The listing builds one solid part. Answer for the finished solid, in the listing's coordinates (mm). Face numbers are marked on the shaded views. A direction names the side the tool comes from. Round coordinates to 2 decimals unless told otherwise and drop trailing zeros. Write each loop counter-clockwise with the first axis right and the second up, starting at its lowest first coordinate (ties: lowest second). Pieces come first, ordered by that corner, then holes. Notation, with made-up numbers: (56, 64) - (61, 64) arc R15 cw to (61, 72) - close; hole circle Ø6 at (-27, 43). An arc over 180 degrees is marked (long way). Use a Markdown table: item, result. Add a question column.
1) A cutting plane is placed at C-C (x = 21). Give the vertices of the cut face in (y, z), then the cut area to 3 significant figures.
2) Each of these flat-tipped pins is pushed along its axis until it touches: P1, Ø2, axis at y = 8, z = -25, coming from the -X side; P2, Ø0.8, axis at y = 8, z = -25, coming from the +X side; P3, Ø6, axis at y = 9.5, z = -23, coming from the -X side. Where does it stop, or does it pass through?
3) Find the intervals of material crossed by probe 1 along Z at (x, y) = (12, 11); probe 2 along X at (y, z) = (10.75, -12); probe 3 along Z at (x, y) = (36.5, 10.75), in increasing order. Write a range as from..to.
4) A cutting plane is placed at B-B (x = 28). Give the vertices of the cut face in (y, z), then the cut area to 3 significant figures.
5) Determine the mould class of the marked faces 4, 5 and 6 for opening direction Z: +Z half, -Z half, draft (parallel to the pull), parting line (faces both ways), or undercut.
6) A cutting plane is placed at D-D (x = -3). Give the vertices of the cut face in (y, z), then the cut area to 3 significant figures.
7) A tool of negligible diameter and unlimited length cuts with its end or side. For the marked faces 1, 2 and 3, from which of +Z, -Z, +X, -X, +Y, -Y can it reach the whole face along a straight path? Write none if from no direction.
8) A cutting plane is placed at A-A (x = 8.5). Give the vertices of the cut face in (y, z), then the cut area to 3 significant figures.
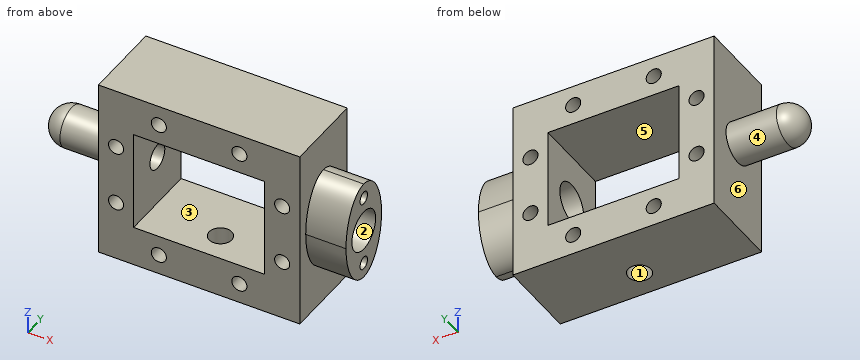
Autodesk Inventor part; units mm, degrees
ref_plane "YZ Plane" through (0, 0, 0) normal (1, 0, 0) x (0, 1, 0)
ref_plane "XZ Plane" through (0, 0, 0) normal (0, 1, 0) x (-1, 0, 0)
ref_plane "XY Plane" through (0, 0, 0) normal (0, 0, 1) x (1, 0, 0)
sketch "Sketch1" plane through (0, 0, 0) normal (0, 1, 0) x (-1, 0, 0)
  line L0 (0, 0) -> (-40, 0)
  line L1 (-40, 0) -> (-40, -36)
  line L2 (-40, -36) -> (0, -36)
  line L3 (0, -36) -> (0, 0)
  line L4 (-7, -28) -> (-33, -28)
  line L5 (-33, -28) -> (-33, -8)
  line L6 (-33, -8) -> (-7, -8)
  line L7 (-7, -8) -> (-7, -28)
  dimension "d0" = 40
  dimension "d1" = 36
  dimension "d2" = 26
extrude "Extrusion1" add sketch "Sketch1" along normal blind 16
sketch "Sketch2" plane through (40, 0, 0) normal (1, 0, 0) x (0, 0, -1)
  line L0 (0, 0) -> (0, 16)
  line L1 (0, 8) -> (8, 8)
  line L2 (28, 0) -> (28, 16)
  line L3 (18, 14) -> (18, 2)
  ellipse E0 centre (18, 8) end of major axis (28, 8) minor radius 6
  line L4 (6.75, 0) -> (6.75, 16)
  line L5 (6.75, 8) -> (9.75, 8)
  circle A0 centre (11, 8) radius 1.25
  circle A1 centre (25, 8) radius 1.25
  circle A2 centre (18, 8) radius 2.5
  line L6 (12.25, 8) -> (15.5, 8)
  line L7 (20.5, 8) -> (23.75, 8)
  line L8 (20.5, 8) -> (23.75, 8)
  line L9 (26.25, 8) -> (28, 8)
  line L10 (8, 8) -> (9.75, 8)
  line L11 (12.25, 8) -> (15.5, 8)
  circle A3 centre (18, 8) radius 4
  line L12 (18, 8) -> (18, 10.5)
  line L13 (18, 12) -> (18, 14)
  dimension "d18" = 8
  dimension "d47" = 10
  dimension "d48" = 6
  dimension "d5" = 8
  dimension "d6" = 20
  dimension "d7" = 6
  dimension "d8" = 12
  dimension "d9" = 3
  dimension "d10" = 14
  dimension "d11" = 2.5
  dimension "d12" = 2.5
  dimension "d13" = 5
  dimension "d49" = 21.25
  dimension "d50" = 28
  dimension "d51" = 0
  dimension "d52" = 0
  dimension "d53" = 0
  dimension "d54" = 28
  dimension "d55" = 8
  dimension "d56" = 8
  dimension "d57" = 1.75
  dimension "d58" = 15.75
  dimension "d59" = 8
  dimension "d60" = 8
  dimension "d61" = 28
  dimension "d62" = 8
extrude "Extrusion3" cut sketch "Sketch2" against normal blind 6 contours A1 | A0
extrude "Extrusion4" cut sketch "Sketch2" against normal blind 40 contours A2 L3 | L3 A2
extrude "Extrusion5" cut sketch "Sketch2" against normal blind 8 contours A3 L7 A2 L3 | L3 A2 L6 A3 | A3 L3 A2 L7 | L6 A2 L3 A3
extrude "Extrusion6" add sketch "Sketch2" along normal blind 8 contours E0 L9 A1 L7 A3 L3 | L3 A3 L6 A0 L5 E0 | E0 L3 A3 L7 A1 L9 | L5 A0 L6 A3 L3 E0
sketch "Sketch3" plane through (0, 0, 0) normal (0, -1, 0) x (1, 0, 0)
  line L0 (0, -20.5) -> (0, -15.5)
  line L1 (0, -18) -> (7, -18)
  line L2 (7, -8) -> (7, -28)
  line L3 (3.5, -18) -> (3.5, -12)
  line L4 (3.5, -12) -> (3.5, -24)
  line L5 (7, -28) -> (7, -36)
  line L6 (40, -36) -> (0, -36)
  line L7 (7, -32) -> (12, -32)
  line L8 (7, -8) -> (7, 0)
  line L9 (7, 0) -> (7, -4)
  line L10 (12, -4) -> (7, -4)
  circle A0 centre (12, -4) radius 1.5
  circle A1 centre (12, -32) radius 1.5
  circle A2 centre (3.5, -24) radius 1.5
  circle A3 centre (3.5, -12) radius 1.5
  line L11 (20, -36) -> (20, 0) construction
  line L12 (0, 0) -> (40, 0) construction
  circle A4 centre (28, -32) radius 1.5
  circle A5 centre (36.5, -24) radius 1.5
  circle A6 centre (36.5, -12) radius 1.5
  circle A7 centre (28, -4) radius 1.5
  dimension "d25" = 6
  dimension "d26" = 12
  dimension "d27" = 5
  dimension "d28" = 3
  dimension "d29" = 3
  dimension "d30" = 3
  dimension "d31" = 3
  dimension "d32" = 90
  dimension "d33" = 32
  dimension "d34" = 4
  dimension "d35" = 18
  dimension "d36" = 36
  dimension "d37" = 13
  dimension "d38" = 16.5
  dimension "d39" = 36
  dimension "d40" = 20
  dimension "d41" = 20
  dimension "d42" = 20
  dimension "d43" = 8
  dimension "d44" = 20.5
extrude "Extrusion7" cut sketch "Sketch3" against normal blind 16
sketch "Sketch4" plane through (0, 0, -36) normal (-1, 0, 0) x (0, 0, 1)
  circle A0 centre (18, 8) radius 4
  point P0 (36, 0)
  dimension "d63" = 8
extrude "Extrusion9" add sketch "Sketch4" along normal blind 14
fillet "Fillet1" radius 4 1 edges at (-14, 8, -22)
sketch "Sketch6" plane through (40, 0, -36) normal (0, 0, -1) x (-1, 0, 0)
  line L0 (33, 5.5) -> (40, 5.5)
  circle A0 centre (19, 5.5) radius 2.25
  point P0 (40, 0)
  dimension "d73" = 4.5
  dimension "d74" = 21
extrude "Extrusion11" cut sketch "Sketch6" against normal blind 10
properties part number "reverse gear steam chest"
Entries:
| question | item | result |
|---|---|---|
| 1 | outline | (0, -36) - (3.25, -36) - (3.25, -28) - (0, -28) - close; (0, -8) - (16, -8) - (16, 0) - (0, 0) - close; (7.75, -36) - (16, -36) - (16, -28) - (7.75, -28) - close |
| 1 | area | 220 mm² |
| 2 | P1 | stops at x = 0 |
| 2 | P2 | stops at x = 34 |
| 2 | P3 | stops at x = -13.33 |
| 3 | probe 1 | z = -36..-33.5, -30.5..-28, -8..-5.5, -2.5..0 |
| 3 | probe 2 | x = 0..2, 5..7, 33..35, 38..48 |
| 3 | probe 3 | z = -36..-25.5, -22.5..-20.9, -15.1..-13.5, -10.5..0 |
| 4 | outline | (0, -36) - (16, -36) - (16, -33.5) - (0, -33.5) - close; (0, -30.5) - (16, -30.5) - (16, -28) - (0, -28) - close; (0, -8) - (16, -8) - (16, -5.5) - (0, -5.5) - close; (0, -2.5) - (16, -2.5) - (16, 0) - (0, 0) - close |
| 4 | area | 160 mm² |
| 5 | face 4 | parting line |
| 5 | face 5 | undercut |
| 5 | face 6 | draft |
| 6 | outline | circle Ø8 at (8, -18) |
| 6 | area | 50.3 mm² |
| 7 | face 1 | -Z |
| 7 | face 2 | +X |
| 7 | face 3 | +Y, -Y |
| 8 | outline | (0, -36) - (16, -36) - (16, -28) - (0, -28) - close; (0, -8) - (16, -8) - (16, 0) - (0, 0) - close |
| 8 | area | 256 mm² |
